Solid Edge part; units mm, degrees
sketch "Sketch1" plane through (0, 0, 0) normal (0, 0, 1) x (1, 0, 0)
  line L0 (-167, -44.5333) -> (167, -44.5333)
  line L1 (167, -44.5333) -> (167, 44.5333)
  line L2 (167, 44.5333) -> (-167, 44.5333)
  line L3 (-167, 44.5333) -> (-167, -44.5333)
extrude "Protrusion1" add sketch "Sketch1" along normal blind 30
sketch "Sketch2" plane through (0, 0, 30) normal (0, 0, 1) x (1, 0, 0)
  line L0 (-152, -25) -> (-91, -25)
  line L1 (-91, -25) -> (-91, 25)
  line L2 (-91, 25) -> (-152, 25)
  line L3 (-152, 25) -> (-152, -25)
extrude "ExtrudedCutout_1" cut sketch "Sketch2" against normal blind 15
fillet "Round_1" radius 3 4 edges at (-152, 25, 22.5) (-91, 25, 22.5) (-152, -25, 22.5) (-91, -25, 22.5)
sketch "Sketch3" plane through (-121.5, 0, 15) normal (0, 0, 1) x (1, 0, 0)
  circle A0 centre (-27.5, 22) radius 2
  circle A1 centre (27.5, 22) radius 2
  circle A2 centre (27.5, -22) radius 2
  circle A3 centre (-27.5, -22) radius 2
extrude "Cutout1" cut sketch "Sketch3" against normal through all
sketch "Sketch4" plane through (0, 0, 0) normal (0, 0, -1) x (-1, 0, 0)
  circle A0 centre (149, 22) radius 4
  circle A1 centre (149, -22) radius 4
  circle A2 centre (94, -22) radius 4
  circle A3 centre (94, 22) radius 4
extrude "ExtrudedCutout_14" cut sketch "Sketch4" against normal blind 5
sketch "Sketch5" plane through (-104.5, 0, 15) normal (0, 0, 1) x (1, 0, 0)
  line L0 (-54.5, 10) -> (263.5, 10)
  line L1 (263.5, 10) -> (263.5, -10)
  line L2 (263.5, -10) -> (-54.5, -10)
  line L3 (-54.5, -10) -> (-54.5, 10)
extrude "ExtrudedCutout_2" cut sketch "Sketch5" against normal blind 6 and the other way blind 6
sketch "Sketch6" plane through (-121.5, -17.5, 15) normal (0, 0, 1) x (-1, 0, 0)
  line L0 (-250.5, 15) -> (-250.5, -50)
  line L1 (-250.5, -50) -> (-280.5, -50)
  line L2 (-280.5, -50) -> (-280.5, 15)
  line L3 (-280.5, 15) -> (-250.5, 15)
extrude "ExtrudedCutout_18" cut sketch "Sketch6" along normal mid plane 20
sketch "Sketch7" plane through (-121.5, -17.5, 15) normal (0, 0, 1) x (-1, 0, 0)
  line L0 (-288.5, -20.5) -> (-280.5, -20.5)
  line L1 (-280.5, -20.5) -> (-280.5, -14.5)
  line L2 (-280.5, -14.5) -> (-288.5, -14.5)
  line L3 (-288.5, -14.5) -> (-288.5, -20.5)
extrude "ExtrudedCutout_19" cut sketch "Sketch7" against normal blind 5
fillet "Round_2" radius 3 6 edges at (-159, 10, 15) (-159, -10, 15) (129, -32.5, 15) (159, -32.5, 15) (159, 32.5, 15) (129, 32.5, 15)
pattern_linear "Pattern1" count 4 spacing 71 along (1, 0, 0) of "ExtrudedCutout_1", "Cutout1", "ExtrudedCutout_14"
fillet "Round1" radius 3 4 edges at (-81, 25, 22.5) (-20, 25, 22.5) (-81, -25, 22.5) (-20, -25, 22.5)
fillet "Round2" radius 3 4 edges at (-10, 25, 22.5) (51, 25, 22.5) (-10, -25, 22.5) (51, -25, 22.5)
fillet "Round3" radius 3 4 edges at (61, 25, 22.5) (122, 25, 22.5) (61, -25, 22.5) (122, -25, 22.5)
sketch "Sketch8" plane through (0, 0, 30) normal (0, 0, 1) x (-1, 0, 0)
  line L0 (-167, 44.5333) -> (167, 44.5333)
  line L1 (167, 44.5333) -> (167, -44.5333)
  line L2 (167, -44.5333) -> (-167, -44.5333)
  line L3 (-167, -44.5333) -> (-167, 44.5333)
extrude "ExtrudedCutout_20" cut sketch "Sketch8" against normal blind 15
fillet "Round_6" radius 6 4 edges at (167, 44.5333, 7.5) (167, -44.5333, 7.5) (-167, 44.5333, 7.5) (-167, -44.5333, 7.5)
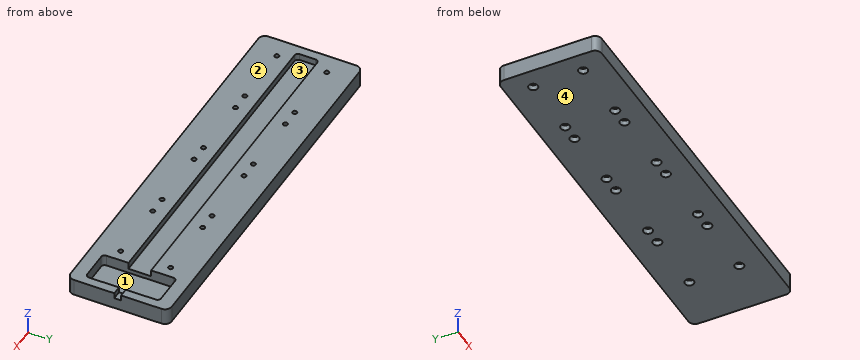
Geometry check sheet. Reference: the model listing, model coordinates, mm. Face numbers are marked on the shaded views. A direction names the side the tool comes from. Give positions to 0.01 mm unless a question says otherwise; leave off trailing zeros. Write each loop counter-clockwise with the first axis right and the second up, starting at its lowest first coordinate (ties: lowest second). Pieces come first, ordered by that corner, then holes. Notation, with made-up numbers: (19, 52.5) - (23, 52.5) arc R23 ccw to (23, 91.5) - close; hole circle Ø2 at (-35.5, 72.5). An arc over 180 degrees is marked (long way). Put each result on its own line as item: value.
1. Go/stop test with flat-tipped pins: pin 1 (2.5 mm diameter, centred on x = 118.5, y = -20, fed in from -Z); pin 2 (2 mm diameter, centred on x = -23.5, y = -8.5, fed in from +Z); pin 3 (1.5 mm diameter, centred on x = 163.5, z = 11.5, fed in from +Y). Record where each tip stops, or that it passes through.
Ans:
pin 1: stops at z = 5
pin 2: stops at z = 9
pin 3: stops at y = 44.27
2. Set-up check for the marked faces 3 and 4: record each of +Z, -Z, +X, -X, +Y, -Y from which the full face is reachable in a straight line by a thin tool's end or side.
Ans:
face 3: +Z
face 4: -Z, +X, -X, +Y, -Y
3. Thickness scan on line 1 (Y direction, x = -7, z = 1.75); line 2 (Y direction, x = -23, z = 8.75); line 3 (Y direction, x = 48, z = 12.5). Record the ranges inside material, lowest first.
Ans:
line 1: y = -44.53 to -26, -18 to 18, 26 to 44.53
line 2: y = -44.53 to -24, -20 to 20, 24 to 44.53
line 3: y = -44.53 to -24, -20 to -10, 10 to 20, 24 to 44.53
4. Draft check along Y on the marked faces 1 and 2. Enter one of: +Y half, -Y half, draft (parallel to the pull), parting line (faces both ways), or undercut.
Ans:
face 1: undercut
face 2: draft
5. Sectioned sample at B-B, the plane y = -13.5. Enter the section's corners in (x, z), plus the area to 3 significant figures.
Ans:
outline: (-167, 0) - (167, 0) - (167, 15) - (159, 15) - (159, 5) - (129, 5) - (129, 15) - (-167, 15) - close
area: 4,710 mm²
6. Sectioned sample at A-A, the plane x = -102.5. Enter the section's corners in (y, z).
Ans:
outline: (-44.53, 0) - (44.53, 0) - (44.53, 15) - (10, 15) - (10, 9) - (-10, 9) - (-10, 15) - (-44.53, 15) - close
